Source: CAD feature listing. Evaluate the final solid. Frame: model axes, mm. A direction names the side the tool comes from. Give positions to 0.01 mm unless a question says otherwise; leave off trailing zeros. Order: outer loops, then holes, each group sorted by start corner. A loop starts at its lowest first (then second) coordinate and runs counter-clockwise, first axis right, second up. Notation, with made-up numbers: (43, 16) -> (56, 16) arc R15 cw to (56, 29) -> close; hole circle Ø8 at (52.5, -38). An arc over 180 degrees is marked (long way). Answer in a Markdown table with one row per item.
```python
from build123d import *

# Parameters (mm, degrees)
F1_DEPTH = 1000
F2_R     = 4
F3_R     = 8


with BuildPart() as f1:
    # F0 (on Top) → F1 (new body)
    with BuildSketch(Plane.XY):
        Polygon((-40, 20), (-40, -20), (40, -20), (40, 20), (33.600028, 20), (30.879981, -14), (-30.879981, -14), (-33.600028, 20), align=None)
    extrude(amount=-F1_DEPTH)

    # F2
    f2_edges = [f1.edges().sort_by_distance(p)[0] for p in [
        (-33.600028, 20, -500),
        (33.600028, 20, -500),
    ]]
    fillet(f2_edges, radius=F2_R)

    # F3
    f3_edges = [f1.edges().sort_by_distance(p)[0] for p in [
        (-30.879981, -14, -500),
        (30.879981, -14, -500),
    ]]
    fillet(f3_edges, radius=F3_R)


solid = f1.part
```
(1) Section query A-A (y = 7.5). Return the cut outline in (x, z).
A:
| item | result |
|---|---|
| outline | (-40, -1000) -> (-32.6, -1000) -> (-32.6, 0) -> (-40, 0) -> close; (32.6, -1000) -> (40, -1000) -> (40, 0) -> (32.6, 0) -> close |
(2) Ray query, probe 1 along X at (y, z) = (7, -473); probe 2 along X at (y, z) = (13, -909); probe 3 along Y at (x, z) = (-8, -587.5). Return the intervals inside material, ascending.
A:
| item | result |
|---|---|
| probe 1 | x = -40 to -32.56, 32.56 to 40 |
| probe 2 | x = -40 to -33.04, 33.04 to 40 |
| probe 3 | y = -20 to -14 |
(3) Pull-direction query (X, two-part tool) for faces 3 (the flat face through (32.4, 5, -493)), 4 (the flat face through (0, -15, 0)), 5 (the flat face through (40, 0, -493)), 6 (the flat face through (-40, 0, -493)); classes: +X half, -X half, draft (parallel to the pull), parting line (faces both ways), or undercut.
A:
| item | result |
|---|---|
| face 3 | undercut |
| face 4 | draft |
| face 5 | +X half |
| face 6 | -X half |
(4) Section query B-B (z = -488). Return the cut outline in (x, y), plus the area to 3 significant figures.
A:
| item | result |
|---|---|
| outline | (-40, -20) -> (40, -20) -> (40, 20) -> (37.29, 20) arc R4 ccw to (33.31, 16.32) -> (31.47, -6.64) arc R8 cw to (23.49, -14) -> (-23.49, -14) arc R8 cw to (-31.47, -6.64) -> (-33.31, 16.32) arc R4 ccw to (-37.29, 20) -> (-40, 20) -> close |
| area | 1,020 mm^2 |
(5) Access query for faces 1 (the flat face through (-32.374, 4.68, -493)), 2 (the flat face through (0, -15, -1000)). Directions: +Z, -Z, +X, -X, +Y, -Y. A direction counts if a zero-diameter tool reaches every point of the face in a straight line with its end or side. Return the directions, or none.
A:
| item | result |
|---|---|
| face 1 | +Z, -Z, +Y |
| face 2 | -Z, +X, -X, +Y, -Y |
(6) Section query C-C (x = -10). Return the cut outline in (y, z).
A:
| item | result |
|---|---|
| outline | (-20, -1000) -> (-14, -1000) -> (-14, 0) -> (-20, 0) -> close |
(7) First-contact query: pin 1 Ø14 at (x, z) = (-4.5, -375) entering from +Y; pin 2 Ø6 at (x, y) = (-10, -10) entering from -Z. Flat tips, straight axial feed; report the tip coordinate or a pass-through.
A:
| item | result |
|---|---|
| pin 1 | stops at y = -14 |
| pin 2 | passes through |
